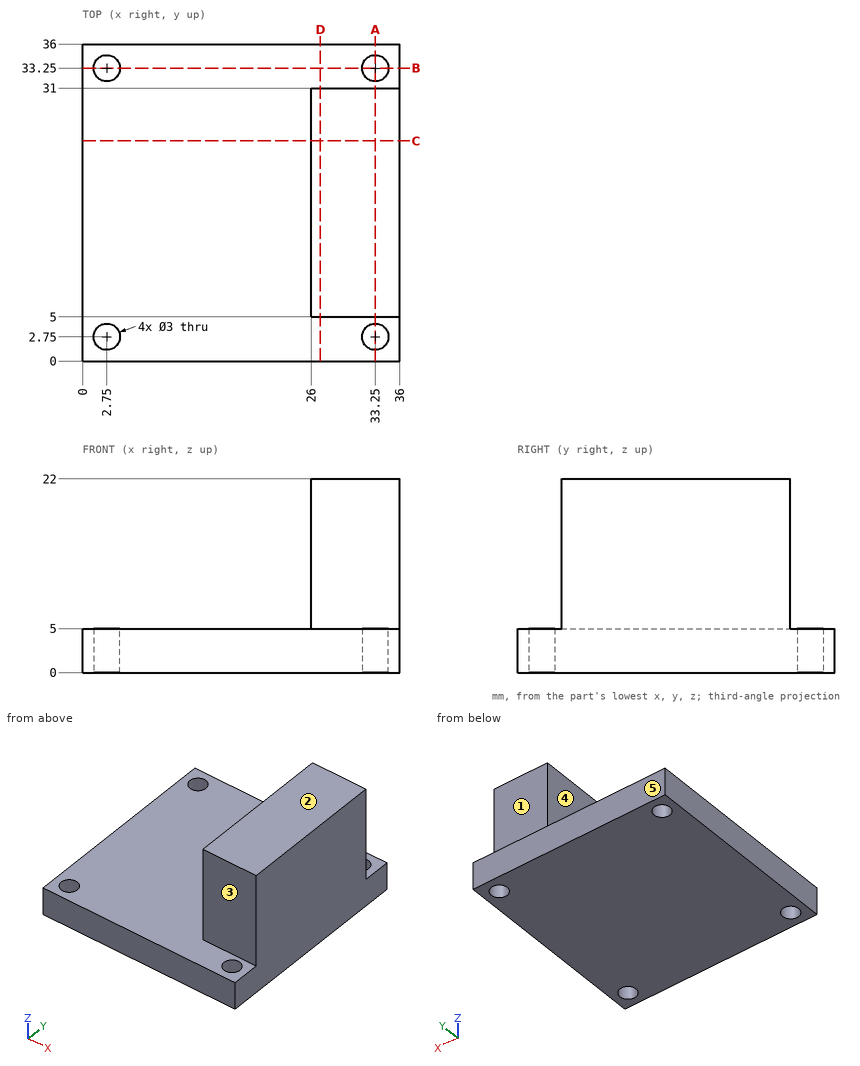
Answer from the drawing. Dimensions are ordinates in mm from the lowest x, y and z of the part. A direction names the side the tool comes from. Give positions to 0.01 mm unless a question says otherwise; leave off trailing zeros. Loops run counter-clockwise (first coordinate to the right, second up) from the corner with the lowest first, then second, coordinate; pieces in that order, holes last. Notation, with made-up numbers: (86.5, -18.75) -> (101.5, -18.75) arc R15 cw to (101.5, -5.75) -> close; hole circle Ø11 at (21, -16.75). An arc over 180 degrees is marked (long way). Answer as CSV lines item,"result".
Item 1: Find section C-C on y = 25. Give the vertices of the cut face in (x, z).
Returned:
outline,"(0, 0) -> (36, 0) -> (36, 22) -> (26, 22) -> (26, 5) -> (0, 5) -> close"
Item 2: Find section B-B on y = 33.25. Give the vertices of the cut face in (x, z).
Returned:
outline,"(0, 0) -> (1.25, 0) -> (1.25, 5) -> (0, 5) -> close; (4.25, 0) -> (31.75, 0) -> (31.75, 5) -> (4.25, 5) -> close; (34.75, 0) -> (36, 0) -> (36, 5) -> (34.75, 5) -> close"
Item 3: For the marked faces 1, 2, 3, 4 and 5, determine the directions among +Z, -Z, +X, -X, +Y, -Y from which every point of the face is accessible in a straight line to the end or side of a thin tool.
Returned:
face 1,"+Z, +X, -X, +Y"
face 2,"+Z, +X, -X, +Y, -Y"
face 3,"+Z, +X, -X, -Y"
face 4,"+Z, -X, +Y, -Y"
face 5,"+Z, -Z, +X, -X, +Y"
Item 4: Find section A-A on x = 33.25. Give the vertices of the cut face in (y, z).
Returned:
outline,"(0, 0) -> (1.25, 0) -> (1.25, 5) -> (0, 5) -> close; (4.25, 0) -> (31.75, 0) -> (31.75, 5) -> (31, 5) -> (31, 22) -> (5, 22) -> (5, 5) -> (4.25, 5) -> close; (34.75, 0) -> (36, 0) -> (36, 5) -> (34.75, 5) -> close"
Item 5: Each of these flat-tipped pins is pushed along its axis until it touches: pin 1 (2.5 mm diameter, centred on x = 33.25, y = 2.75, fed in from -Z); pin 2 (10 mm diameter, centred on x = 12, y = 13.5, fed in from +Z); pin 3 (5 mm diameter, centred on x = 32, z = 11, fed in from +Y); pin 4 (10 mm diameter, centred on y = 14.5, z = 16.5, fed in from -X). Where does it stop, or does it pass through?
Returned:
pin 1,"passes through"
pin 2,"stops at z = 5"
pin 3,"stops at y = 31"
pin 4,"stops at x = 26"
Item 6: Consider line 1 (X direction, y = 2.75, z = 3.25); line 2 (Z direction, x = 13.5, y = 17.5). Determine where each line is inside the solid, lowest interval first. Write a range as [from, to].
Returned:
line 1,"x = [0, 1.25], [4.25, 31.75], [34.75, 36]"
line 2,"z = [0, 5]"
Item 7: Find section D-D on x = 27. Give the vertices of the cut face in (y, z), plus the area to 3 significant figures.
Returned:
outline,"(0, 0) -> (36, 0) -> (36, 5) -> (31, 5) -> (31, 22) -> (5, 22) -> (5, 5) -> (0, 5) -> close"
area,"622 mm²"
